Part model, mm, in its own coordinate system. Round coordinates to 2 decimals unless told otherwise and drop trailing zeros. Loops run counter-clockwise (first coordinate to the right, second up) from the corner with the lowest first, then second, coordinate; pieces in that order, holes last. Notation, with made-up numbers: (81, 38.25) -> (132, 38.25) arc R12 cw to (132, 57.25) -> close; hole circle Ø6 at (-25.5, -5). An arc over 180 degrees is marked (long way). Use a Markdown table: item, result. Add a question column.
Item 1: Probe line 1 (Y direction, x = 240, z = 4.6); line 2 (X direction, y = 63, z = 0.5). List the from-to ranges inside material, lowest first. Write a range as [from, to].
Item 2: Flat gauge pins, fed straight in: pin 1 (2.5 mm diameter, centred on x = 273.5, z = 1.5, fed in from -Y); pin 2 (2 mm diameter, centred on x = 128, y = 58, fed in from -Z); pin 3 (1 mm diameter, centred on y = 70, z = 4.5, fed in from -X); pin 4 (2.5 mm diameter, centred on y = -1.5, z = 3, fed in from -X). Where does each tip first touch, or does it go through?
Item 3: Cut at A-A, the plane x = 534.5. List the corners of the cut face in (y, z), plus the area to 3 significant figures.
```python
from build123d import *

# Parameters (mm, degrees)
CROQUIS1_W              = 780
CROQUIS1_H              = 145
CROQUIS1_W_2            = 150
CROQUIS1_H_2            = 5
CROQUIS1_W_3            = 5
CROQUIS1_H_3            = 35
SALIENTE_EXTRUIR1_DEPTH = 5
CORTAR_EXTRUIR1_DEPTH   = 10


with BuildPart() as part:
    # Croquis1 → Saliente-Extruir1 (new body)
    with BuildSketch(Plane.XY):
        with Locations((390, 72.5)):
            Rectangle(CROQUIS1_W, CROQUIS1_H)
        with Locations((622.5, -2.5)):
            Rectangle(CROQUIS1_W_2, CROQUIS1_H_2)
        Polygon((390, 0), (315, 0), (315, -5), (465, -5), (465, 0), align=None)
        with Locations((157.5, -2.5)):
            Rectangle(CROQUIS1_W_2, CROQUIS1_H_2)
        with Locations((-2.5, 36.25)):
            Rectangle(CROQUIS1_W_3, CROQUIS1_H_3)
        with Locations((782.5, 36.25)):
            Rectangle(CROQUIS1_W_3, CROQUIS1_H_3)
        with Locations((782.5, 108.75)):
            Rectangle(CROQUIS1_W_3, CROQUIS1_H_3)
        with Locations((-2.5, 108.75)):
            Rectangle(CROQUIS1_W_3, CROQUIS1_H_3)
    extrude(amount=SALIENTE_EXTRUIR1_DEPTH)

    # Croquis2 → Cortar-Extruir1 (cut)
    with BuildSketch(Plane.XY.offset(5)):
        Polygon((275.35, 0), (272.15, 0), (272.15, 5), (270.35, 5), (270.35, 8.2), (272.15, 8.2), (272.15, 17.2), (275.35, 17.2), (275.35, 8.2), (277.15, 8.2), (277.15, 5), (275.35, 5), align=None)
        Polygon((507.85, 8.2), (507.85, 17.2), (504.65, 17.2), (504.65, 8.2), (502.85, 8.2), (502.85, 5), (504.65, 5), (504.65, 0), (507.85, 0), (507.85, 5), (509.65, 5), (509.65, 8.2), align=None)
    extrude(amount=-CORTAR_EXTRUIR1_DEPTH, mode=Mode.SUBTRACT)


solid = part.part
```
A:
| question | item | result |
|---|---|---|
| 1 | line 1 | y = [0, 145] |
| 1 | line 2 | x = [0, 780] |
| 2 | pin 1 | stops at y = 17.2 |
| 2 | pin 2 | stops at z = 0 |
| 2 | pin 3 | stops at x = 0 |
| 2 | pin 4 | stops at x = 82.5 |
| 3 | outline | (0, 0) -> (145, 0) -> (145, 5) -> (0, 5) -> close |
| 3 | area | 725 mm^2 |
